```python
from build123d import *

# Parameters (mm, degrees)
F1_DEPTH  = 66
F2_R      = 1.5
F3_DEPTH  = 25
F4_R      = 1
F5_DEPTH  = 25
F6_R      = 5
F7_R      = 6.5
F8_W      = 7
F8_H      = 48
F9_DEPTH  = 100
F11_DEPTH = 66


with BuildPart() as f1:
    # F0 (on Top) → F1 (new body)
    with BuildSketch(Plane.XY):
        with BuildLine():
            Line((54.5, 33), (54.5, -26.488032))
            Line((54.5, -26.488032), (53.5, -29.23551))
            Line((53.5, -29.23551), (53.5, -31.5))
            Line((53.5, -31.5), (55, -31.5))
            Line((55, -31.5), (55, -29.5))
            Line((55, -29.5), (56, -26.752523))
            Line((56, -26.752523), (56, 33))
            ThreePointArc((56, 33), (54.535534, 36.535534), (51, 38))
            Line((51, 38), (-42.5, 38))
            ThreePointArc((-42.5, 38), (-46.035534, 36.535534), (-47.5, 33))
            Line((-47.5, 33), (-47.5, 0))
            Line((-47.5, 0), (-46, 0))
            Line((-46, 0), (-46, 33))
            ThreePointArc((-46, 33), (-44.974874, 35.474874), (-42.5, 36.5))
            Line((-42.5, 36.5), (51, 36.5))
            ThreePointArc((51, 36.5), (53.474874, 35.474874), (54.5, 33))
        make_face()
    extrude(amount=F1_DEPTH)

    # F2 (on face) → F3 (cut)
    with BuildSketch(Plane(origin=(0, 38, 0), x_dir=(-1, 0, 0), z_dir=(0, 1, 0))):
        with Locations((-38.75, 58)):
            Circle(F2_R)
        with Locations((-38.75, 8)):
            Circle(F2_R)
        with Locations((38.75, 8)):
            Circle(F2_R)
        with Locations((38.75, 58)):
            Circle(F2_R)
    extrude(amount=-F3_DEPTH, mode=Mode.SUBTRACT)

    # F4 (on face) → F5 (cut)
    with BuildSketch(Plane.YZ.offset(56)):
        with BuildLine():
            Line((-17, 58), (-21, 58))
            ThreePointArc((-21, 58), (-23.12132, 57.12132), (-24, 55))
            Line((-24, 55), (-24, 11))
            ThreePointArc((-24, 11), (-23.12132, 8.87868), (-21, 8))
            Line((-21, 8), (-17, 8))
            ThreePointArc((-17, 8), (-14.87868, 8.87868), (-14, 11))
            Line((-14, 11), (-14, 55))
            ThreePointArc((-14, 55), (-14.87868, 57.12132), (-17, 58))
        make_face()
        with BuildLine():
            Line((24, 58), (-5, 58))
            ThreePointArc((-5, 58), (-7.12132, 57.12132), (-8, 55))
            Line((-8, 55), (-8, 11))
            ThreePointArc((-8, 11), (-7.12132, 8.87868), (-5, 8))
            Line((-5, 8), (24, 8))
            ThreePointArc((24, 8), (26.12132, 8.87868), (27, 11))
            Line((27, 11), (27, 55))
            ThreePointArc((27, 55), (26.12132, 57.12132), (24, 58))
        make_face()
        with Locations((-19, 61)):
            Circle(F4_R)
        with Locations((9.5, 61)):
            Circle(F4_R)
        with Locations((9.5, 5)):
            Circle(F4_R)
        with Locations((-19, 5)):
            Circle(F4_R)
    extrude(amount=-F5_DEPTH, mode=Mode.SUBTRACT)

    # F6
    f6_edges = [f1.edges().sort_by_distance(p)[0] for p in [
        (55, -29.5, 33),
        (54.5, -26.488032, 33),
    ]]
    fillet(f6_edges, radius=F6_R)

    # F7
    f7_edges = [f1.edges().sort_by_distance(p)[0] for p in [
        (56, -26.752523, 33),
        (53.5, -29.23551, 33),
    ]]
    fillet(f7_edges, radius=F7_R)

    # F8 (on Top) → F9 (cut)
    with BuildSketch(Plane.XY):
        with Locations((-46, 19)):
            Rectangle(F8_W, F8_H)
    extrude(amount=F9_DEPTH, mode=Mode.SUBTRACT)

    # F10 (on Top) → F11 (join)
    with BuildSketch(Plane.XY):
        with BuildLine():
            Line((-48.496257, 37), (-48.496257, 35.5))
            Line((-48.496257, 35.5), (-46.746257, 35.5))
            ThreePointArc((-46.746257, 35.5), (-45.878016, 35.575961), (-45.036156, 35.801537))
            Line((-45.036156, 35.801537), (-43.697071, 36.288924))
            ThreePointArc((-43.697071, 36.288924), (-43.107769, 36.446827), (-42.5, 36.5))
            Line((-42.5, 36.5), (-42.5, 38))
            ThreePointArc((-42.5, 38), (-43.368241, 37.924039), (-44.210101, 37.698463))
            Line((-44.210101, 37.698463), (-45.549186, 37.211076))
            ThreePointArc((-45.549186, 37.211076), (-46.138488, 37.053173), (-46.746257, 37))
            Line((-46.746257, 37), (-48.496257, 37))
        make_face()
    extrude(amount=F11_DEPTH)


solid = f1.part
```
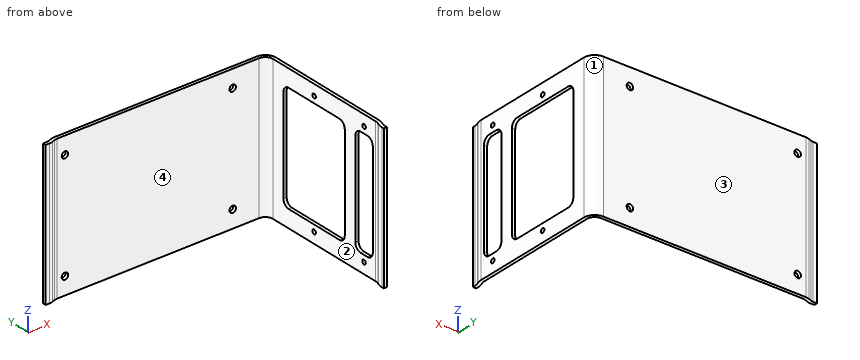
Source: CAD feature listing. Evaluate the final solid. Frame: model axes, mm. Face numbers are marked on the shaded views. Coordinates: 2 decimals unless noted, no trailing zeros. Order: outer loops, then holes, each group sorted by start corner. A loop starts at its lowest first (then second) coordinate and runs counter-clockwise, first axis right, second up. Notation, with made-up numbers: M -22.5,42.25 L -11.5,42.25 A38 ccw -11.5,80.25 Z; hole C 13.5,49.25 d5. An arc over 180 degrees is marked long. Write each question's results on one line, items separated by ' | '. Start each with the question number.
1) Section query B-B (z = 13). Give the number of separate pieces and of enclosed holes in the cut face, plus the area to 3 significant figures.
2) Line query: line 1 (Z direction, x = -38.75, y = 37.25); line 2 (Z direction, x = 55.2, y = 9.5); line 3 (Y direction, x = 1.5, z = 11). Output: solid intervals per line, ascending. Write a range as from..to.
3) Draft query along X for the marked faces 1, 2, 3 and 4. Return one class per face: released by +X, released by -X, zero draft, split by the parting line, or undercut.
4) Contact query for flat-ended pins moving along their axis: pin 1 Ø2 at (y, z) = (30.5, 56.5) entering from -X; pin 2 Ø8 at (x, z) = (31, 37) entering from -Y; pin 3 Ø1.4 at (x, z) = (-47.5, 41.5) entering from +Y. Output: stop coordinate, or through.
5) Section query D-D (x = 11.5). Return the cut outline in (y, z).
6) Section query C-C (y = -15.5). Return the cut outline in (x, z).
7) Section query A-A (x = -38.75). Return the cut outline in (y, z), plus the area to 3 significant figures.
Answers:
1) separate pieces: 3 | enclosed holes: 0 | area: 189 mm^2
2) line 1: z = 0..6.5, 9.5..56.5, 59.5..66 | line 2: z = 0..4, 6..8, 58..60, 62..66 | line 3: y = 36.5..38
3) face 1: released by +X | face 2: released by -X | face 3: zero draft | face 4: undercut
4) pin 1: stops at x = 54.5 | pin 2: stops at y = 36.5 | pin 3: stops at y = 37
5) outline: M 36.5,0 L 38,0 L 38,66 L 36.5,66 Z
6) outline: M 54.5,0 L 56,0 L 56,8.4 L 54.5,8.4 Z; M 54.5,57.6 L 56,57.6 L 56,66 L 54.5,66 Z
7) outline: M 36.5,0 L 38,0 L 38,6.5 L 36.5,6.5 Z; M 36.5,9.5 L 38,9.5 L 38,56.5 L 36.5,56.5 Z; M 36.5,59.5 L 38,59.5 L 38,66 L 36.5,66 Z | area: 90.0 mm^2
